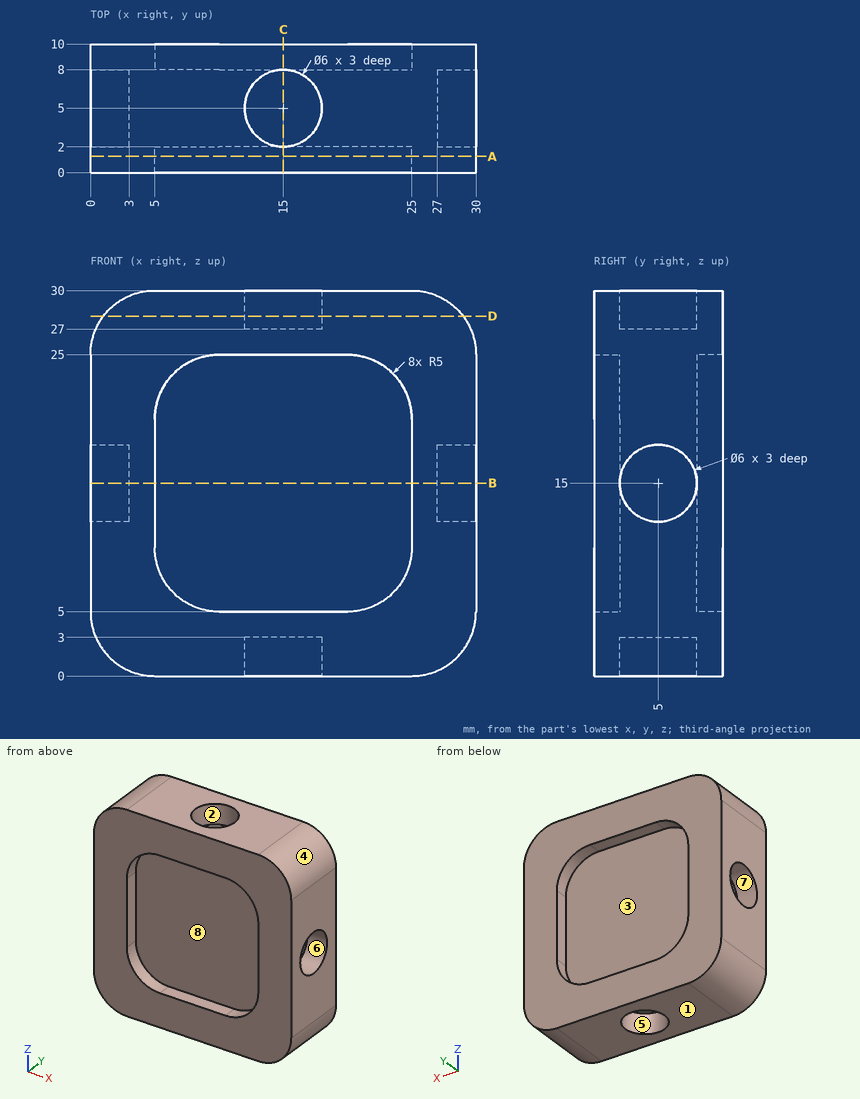
The figure shows three views and two pictorial views of one solid part (mm, origin at its lowest corner). Answer the questions. A direction names the side the tool comes from. Round coordinates to 2 decimals unless told otherwise and drop trailing zeros. Order: outer loops, then holes, each group sorted by start corner. A loop starts at its lowest first (then second) coordinate and runs counter-clockwise, first axis right, second up. Notation, with made-up numbers: (1, 57) -> (8, 57) arc R21 cw to (8, 62) -> close; hole circle Ø3 at (-32, -26). An arc over 180 degrees is marked (long way). One line per item, written item: value.
Item 1: Find section D-D, the plane z = 28. Give the vertices of the cut face in (x, y), then the cut area to 3 significant figures.
Taken from the geometry:
outline: (1, 0) -> (29, 0) -> (29, 10) -> (1, 10) -> close; hole circle Ø6 at (15, 5)
area: 252 mm2
Item 2: Find section A-A, the plane y = 1.25. Give the vertices of the cut face in (x, z), then the cut area to 3 significant figures.
Taken from the geometry:
outline: (0, 5) arc R5 ccw to (5, 0) -> (25, 0) arc R5 ccw to (30, 5) -> (30, 25) arc R5 ccw to (25, 30) -> (5, 30) arc R5 ccw to (0, 25) -> close; hole (5, 10) arc R5 ccw to (10, 5) -> (20, 5) arc R5 ccw to (25, 10) -> (25, 20) arc R5 ccw to (20, 25) -> (10, 25) arc R5 ccw to (5, 20) -> close
area: 500 mm2
Item 3: For the marked faces 5, 6, 7 and 8, determine the directions among +Z, -Z, +X, -X, +Y, -Y from which every point of the face is accessible in a straight line to the end or side of a thin tool.
Taken from the geometry:
face 5: -Z
face 6: +X
face 7: -X
face 8: -Y
Item 4: For a pull along Z with two mould halves and no side action, classify the marked faces 1, 2, 3 and 4 as released by +Z, released by -Z, zero draft, split by the parting line, or undercut.
Taken from the geometry:
face 1: released by -Z
face 2: zero draft
face 3: undercut
face 4: released by +Z
Item 5: Straight lines are drawn through the part: L1, parallel to Z at x = 16.75, y = 1; L2, parallel to Y at x = 15, z = 2.3. For each, find the intervals that lie inside material, in ascending order.
Taken from the geometry:
L1: z = 0 to 5, 25 to 30
L2: y = 0 to 2, 8 to 10
Item 6: Find section C-C, the plane x = 15. Give the vertices of the cut face in (y, z), then the cut area to 3 significant figures.
Taken from the geometry:
outline: (0, 0) -> (2, 0) -> (2, 3) -> (8, 3) -> (8, 0) -> (10, 0) -> (10, 5) -> (8, 5) -> (8, 25) -> (10, 25) -> (10, 30) -> (8, 30) -> (8, 27) -> (2, 27) -> (2, 30) -> (0, 30) -> (0, 25) -> (2, 25) -> (2, 5) -> (0, 5) -> close
area: 184 mm2
Item 7: Given P1, Ø3, axis at x = 14.5, y = 5, coming from the +Z side; P2, Ø1.8, axis at x = 15.5, y = 6.5, coming from the -Z side; P3, Ø1.5, axis at x = 23.5, z = 15.5, coming from the +Y side, each flat-ended and moving along its own axis, determine where each tip first touches the part or whether it passes through.
Taken from the geometry:
P1: stops at z = 27
P2: stops at z = 3
P3: stops at y = 8
Item 8: Find section B-B, the plane z = 15. Give the vertices of the cut face in (x, y), then the cut area to 3 significant figures.
Taken from the geometry:
outline: (0, 0) -> (5, 0) -> (5, 2) -> (25, 2) -> (25, 0) -> (30, 0) -> (30, 2) -> (27, 2) -> (27, 8) -> (30, 8) -> (30, 10) -> (25, 10) -> (25, 8) -> (5, 8) -> (5, 10) -> (0, 10) -> (0, 8) -> (3, 8) -> (3, 2) -> (0, 2) -> close
area: 184 mm2
